The figure shows three views and two pictorial views of one solid part (mm, origin at its lowest corner). Answer the questions. A direction names the side the tool comes from. Coordinates: 2 decimals unless noted, no trailing zeros. Loops run counter-clockwise (first coordinate to the right, second up) from the corner with the lowest first, then second, coordinate; pieces in that order, holes last. Notation, with made-up numbers: (89, 15) -> (95, 15) arc R22 ccw to (95, 42) -> close; hole circle Ø11 at (-18, 22). An arc over 180 degrees is marked (long way). Answer as a JSON object with one key per item and string values. Group by question number.
1) Section D-D, the plane z = 19.25 is taken. Give the vertices of the cut face in (x, y), plus the area to 3 significant figures.
2) Determine the mould class of the marked faces 3, 4, 5 and 6 for opening direction Z: released by +Z, released by -Z, zero draft, split by the parting line, or undercut.
3) Consider probe 1 along X at (y, z) = (24.25, 22); probe 2 along Y at (x, z) = (2.75, 12.5); probe 3 along Y at (x, z) = (11, 6.5). Determine where each line is inside the solid, lowest interval first. Write a range as [from, to].
4) Flat-ended cylindrical pins translate along their axes: P1, Ø8, axis at x = 9.5, z = 7, coming from the +Y side; P2, Ø2, axis at y = 21, z = 22, coming from the +X side; P3, Ø4, axis at x = 12.5, z = 15, coming from the +Y side. Find the tip coordinate at first contact, or state that the pin passes through.
5) Section A-A, the plane z = 12.5 is taken. Give the vertices of the cut face in (x, y).
6) Section B-B, the plane y = 19.75 is taken. Give the vertices of the cut face in (x, z), plus the area to 3 significant figures.
7) Which of the six approach directions +Z, -Z, +X, -X, +Y, -Y give full straight-line access (tool end or side, diameter ignored) to the marked faces 1 and 2?
8) Section C-C, the plane x = 6.5 is taken. Give the vertices of the cut face in (y, z).
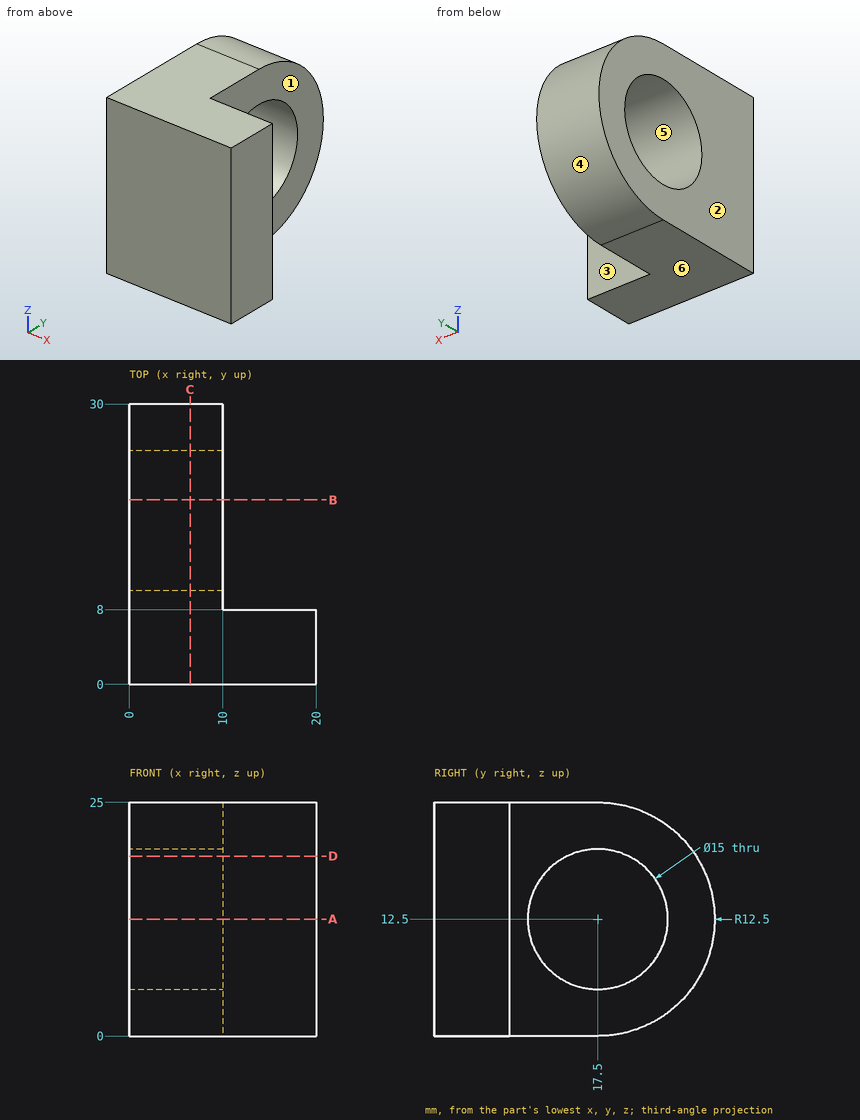
Determined:
{
 "1": {"outline": "(0, 0) -> (20, 0) -> (20, 8) -> (10, 8) -> (10, 14.23) -> (0, 14.23) -> close; (0, 20.77) -> (10, 20.77) -> (10, 28.02) -> (0, 28.02) -> close", "area": "295 mm²"},
 "2": {"face 3": "zero draft", "face 4": "split by the parting line", "face 5": "undercut", "face 6": "released by -Z"},
 "3": {"probe 1": "[0, 10]", "probe 2": "[0, 10], [25, 30]", "probe 3": "[0, 8]"},
 "4": {"P1": "y = 29.91", "P2": "x = 10", "P3": "y = 8"},
 "5": {"outline": "(0, 0) -> (20, 0) -> (20, 8) -> (10, 8) -> (10, 10) -> (0, 10) -> close; (0, 25) -> (10, 25) -> (10, 30) -> (0, 30) -> close"},
 "6": {"outline": "(0, 0.2) -> (10, 0.2) -> (10, 5.35) -> (0, 5.35) -> close; (0, 19.65) -> (10, 19.65) -> (10, 24.8) -> (0, 24.8) -> close", "area": "103 mm²"},
 "7": {"face 1": "+Z, -Z, +X, +Y", "face 2": "+Z, -Z, -X, +Y, -Y"},
 "8": {"outline": "(0, 0) -> (17.5, 0) arc R12.5 ccw to (17.5, 25) -> (0, 25) -> close; hole circle Ø15 at (17.5, 12.5)"}
}
